Can you work these out from the model? Positions are in its coordinate system, mm. Give positions to 0.01 mm unless a question says otherwise; leave off trailing zeros. Loops run counter-clockwise (first coordinate to the right, second up) from the corner with the lowest first, then second, coordinate; pieces in that order, holes last. Notation, with made-up numbers: M 39.5,59 L 62.5,59 A31 ccw 62.5,84 Z; hole C -25.75,-1.5 d2. An arc over 180 degrees is marked long. Use CSV: the item, a comma, the result in double quotes.
Autodesk Inventor part; units mm, degrees
ref_plane "YZ Plane" through (0, 0, 0) normal (1, 0, 0) x (0, 1, 0)
ref_plane "XZ Plane" through (0, 0, 0) normal (0, 1, 0) x (-1, 0, 0)
ref_plane "XY Plane" through (0, 0, 0) normal (0, 0, 1) x (1, 0, 0)
sketch "Sketch1" plane through (0, 0, 0) normal (1, 0, 0) x (0, 1, 0)
  line L0 (0, 0) -> (12.7, 0)
  line L1 (12.7, 0) -> (12.7, -50.8)
  line L2 (12.7, -50.8) -> (0, -50.8)
  line L3 (0, -50.8) -> (0, 0)
  arc A0 (12.7, 9.525) -> (1.6567, 10.3991) centre (7.1437, 9.525) ccw
  line L4 (12.7, 0) -> (12.7, 9.525)
  line L5 (1.6567, 10.3991) -> (0, 0)
  line L6 (7.1437, 9.525) -> (7.1437, 0) construction
  circle A1 centre (7.1437, 9.525) radius 6.35 construction
  line L7 (12.7, -25.4) -> (0, -25.4) construction
  arc A2 (1.6567, -61.1991) -> (12.7, -60.325) centre (7.1438, -60.325) ccw
  line L8 (12.7, -50.8) -> (12.7, -60.325)
  line L9 (1.6567, -61.1991) -> (0, -50.8)
  circle A3 centre (7.1437, 9.525) radius 2.3813
  circle A4 centre (7.1438, -60.325) radius 2.3813
  dimension "d0" = 12.7
  dimension "d1" = 50.8
  dimension "d7" = 12.7
  dimension "d8" = 9.525
  dimension "d11" = 4.7625
  dimension "d25" = 3.175
extrude "Extrusion1" add sketch "Sketch1" along normal blind 3.175
sketch "Sketch2" plane through (3.175, 0, 0) normal (1, 0, 0) x (0, 0, -1)
  line L0 (60.325, 12.7) -> (-9.525, 12.7)
  line L1 (25.4, 12.7) -> (25.4, 0) construction
  line L2 (0, 0) -> (50.8, 0)
  line L3 (0, 12.7) -> (50.8, 12.7) construction
  line L4 (50.8, 12.7) -> (50.8, 38.1) construction
  line L5 (50.8, 38.1) -> (0, 38.1) construction
  line L6 (0, 38.1) -> (0, 12.7) construction
  line L7 (3.175, 34.925) -> (47.625, 34.925) construction
  line L8 (47.625, 34.925) -> (47.625, 15.875) construction
  line L9 (47.625, 15.875) -> (3.175, 15.875) construction
  line L10 (3.175, 15.875) -> (3.175, 34.925) construction
  circle A0 centre (9.525, 6.35) radius 2.667
  line L11 (25.4, 6.35) -> (44.9012, 6.35) construction
  circle A1 centre (25.4, 6.35) radius 2.667
  line L12 (9.525, 6.35) -> (32.9122, 6.35) construction
  circle A2 centre (41.275, 6.35) radius 2.667
  circle A3 centre (9.525, 6.35) radius 2.667
  circle A4 centre (25.4, 6.35) radius 2.667
  circle A5 centre (41.275, 6.35) radius 2.667
  dimension "d16" = 50.8
  dimension "d17" = 25.4
  dimension "d18" = 3.175
  dimension "d19" = 5.334
  dimension "d20" = 15.875
  dimension "d21" = 6.35
  dimension "d22" = 5.334
extrude "Extrusion2" cut sketch "Sketch2" against normal through all
fillet "Fillet1" radius 3.175 2 edges at (1.5875, 0, 0) (1.5875, 0, -50.8)
properties part number "ElevatorCarriageBearingGusset"
Q1. I want a section at C-C, the plane y = 1. Please give me the cut outline in (x, z) (3 decimals).
Model answer:
outline,"M 0,-57.077 L 3.175,-57.077 L 3.175,6.277 L 0,6.277 Z"
Q2. If we mould it in two halves opening along Y, with no side actions, what happens to faces 1 (the flat face through (3.175, 3, -25)), 2 (the cylindrical face through (1.61, 7.151, -27.944)), 3 (the cylindrical face through (1.57, 7.47, 15.07))? For each: released by +Y, released by -Y, zero draft, split by the parting line, or undercut.
Model answer:
face 1,"zero draft"
face 2,"undercut"
face 3,"split by the parting line"
Q3. I want a section at B-B, the plane y = 6.35. Please give me the cut outline in (x, z) (3 decimals).
Model answer:
outline,"M 0,-65.824 L 3.175,-65.824 L 3.175,-62.57 L 0,-62.57 Z; M 0,-58.08 L 3.175,-58.08 L 3.175,-43.942 L 0,-43.942 Z; M 0,-38.608 L 3.175,-38.608 L 3.175,-28.067 L 0,-28.067 Z; M 0,-22.733 L 3.175,-22.733 L 3.175,-12.192 L 0,-12.192 Z; M 0,-6.858 L 3.175,-6.858 L 3.175,7.28 L 0,7.28 Z; M 0,11.77 L 3.175,11.77 L 3.175,15.024 L 0,15.024 Z"
Q4. I want a section at D-D, the plane z = 2.5. Please give me the cut outline in (x, y) (3 decimals), then the cut area to 3 significant figures.
Model answer:
outline,"M 0,0.398 L 3.175,0.398 L 3.175,12.7 L 0,12.7 Z"
area,"39.1 mm2"
Q5. Please list where these lines run through material, in increasing order: L1, parallel to Z at x = 1.45, y = 5.75; L2, parallel to Y at x = 2.3, z = -25.4; L3, parallel to Y at x = 0.5, z = -58.5. Write a range as from..to.
Model answer:
L1,"-65.7..-62.26, -58.39..-43.87, -38.68..-28, -22.8..-12.12, -6.93..7.59, 11.46..14.9"
L2,"0..3.68, 9.02..12.7"
L3,"1.23..5.61, 8.67..12.7"
Q6. I want a section at A-A, the plane x = 1.45. Please give me the cut outline in (y, z) (3 decimals).
Model answer:
outline,"M 0,-50.549 A3.175 ccw 0.04,-51.048 L 1.657,-61.199 A5.556 ccw 12.7,-60.325 L 12.7,9.525 A5.556 ccw 1.657,10.399 L 0.04,0.248 A3.175 ccw 0,-0.251 Z; hole C 6.35,-41.275 d5.334; hole C 6.35,-25.4 d5.334; hole C 6.35,-9.525 d5.334; hole C 7.144,-60.325 d4.763; hole C 7.144,9.525 d4.763"
